For this review, use the dimensioned drawing (mm, ordinates from the lowest corner) and the shaded views. A direction names the side the tool comes from. Coordinates: 2 decimals unless noted, no trailing zeros. Loops run counter-clockwise (first coordinate to the right, second up) from the corner with the lowest first, then second, coordinate; pieces in that order, holes last. Notation, with made-up numbers: M 84.25,10.5 L 120.25,10.5 A18 cw 120.25,35.5 Z; hole C -2,17.5 d2. An arc over 180 degrees is marked long. Write item = value, one per line.
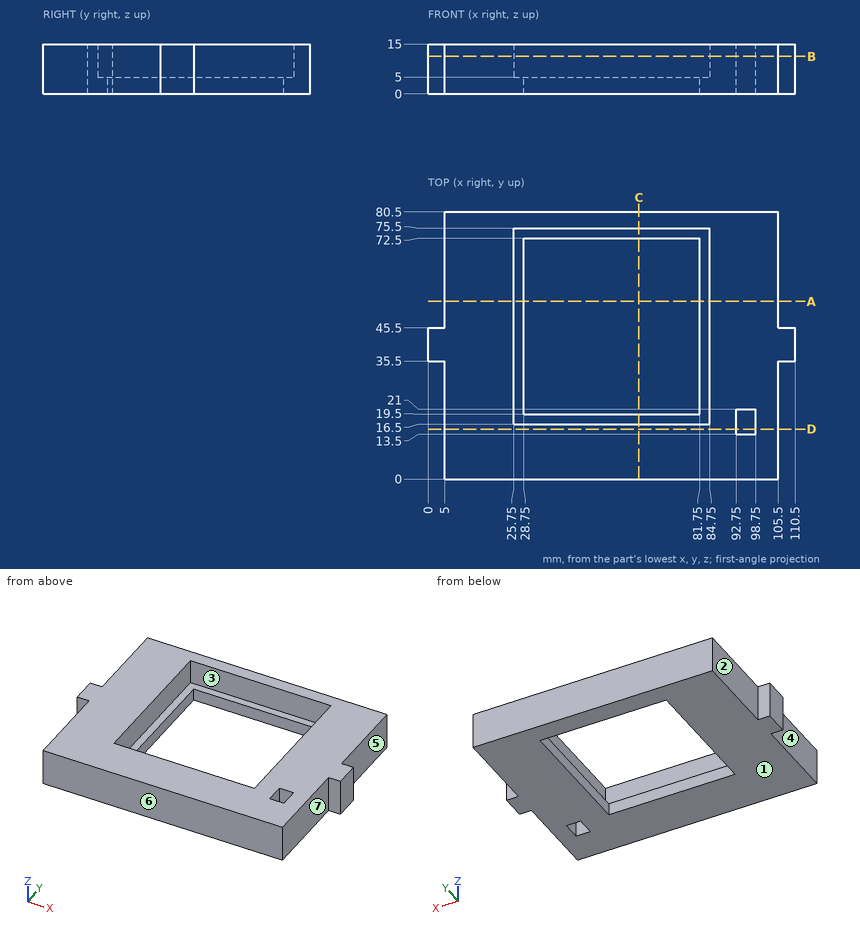
Q1. For pin 1 Ø4 at (x, z) = (1.5, 10.5) entering from -Y; pin 2 Ø5 at (y, z) = (53.5, 8) entering from +X; pin 3 Ø4 at (x, z) = (108.5, 8.5) entering from +Y, all flat-tipped, find the tip position at first contact; note any pin that passes through.
Solved:
pin_1 = 35.5
pin_2 = 105.5
pin_3 = 45.5
Q2. Machinability: for the marked faces 4, 5, 6 and 7, which of the approach directions +Z, -Z, +X, -X, +Y, -Y give a long, thin tool a straight path to every point of the face, cutting with its end or side? Answer none if there is none.
Solved:
face_4 = +Z, -Z, -X, -Y
face_5 = +Z, -Z, +X, +Y
face_6 = +Z, -Z, +X, -X, -Y
face_7 = +Z, -Z, +X, -Y
Q3. Add section B-B (z = 11.25). Write out the cut boundary in (x, y), and give its area (3 significant figures).
Solved:
outline = M 0,35.5 L 5,35.5 L 5,0 L 105.5,0 L 105.5,35.5 L 110.5,35.5 L 110.5,45.5 L 105.5,45.5 L 105.5,80.5 L 5,80.5 L 5,45.5 L 0,45.5 Z; hole M 25.75,16.5 L 84.75,16.5 L 84.75,75.5 L 25.75,75.5 Z; hole M 92.75,13.5 L 98.75,13.5 L 98.75,21 L 92.75,21 Z
area = 4,660 mm²
Q4. Add section C-C (x = 63.5). Write out the cut boundary in (y, z), and give its area (4 significant figures).
Solved:
outline = M 0,0 L 19.5,0 L 19.5,5 L 16.5,5 L 16.5,15 L 0,15 Z; M 72.5,0 L 80.5,0 L 80.5,15 L 75.5,15 L 75.5,5 L 72.5,5 Z
area = 352.5 mm²
Q5. For line 1 along Y through (x, z) = (37.5, 2.75); line 2 along Y through (x, z) = (41, 11); line 3 along X through (y, z) = (38, 12), list the stretches that pass through material, from the lowest coordinate up.
Solved:
line_1 = 0 to 19.5, 72.5 to 80.5
line_2 = 0 to 16.5, 75.5 to 80.5
line_3 = 0 to 25.75, 84.75 to 110.5
Q6. Add section A-A (y = 53.5). Write out the cut boundary in (x, z), and give its area (4 significant figures).
Solved:
outline = M 5,0 L 28.75,0 L 28.75,5 L 25.75,5 L 25.75,15 L 5,15 Z; M 81.75,0 L 105.5,0 L 105.5,15 L 84.75,15 L 84.75,5 L 81.75,5 Z
area = 652.5 mm²
Q7. Draft analysis for pull direction X (two halves, no side actions). For the marked faces 1, 2 and 3, state which applies: +X half, -X half, draft (parallel to the pull), parting line (faces both ways), or undercut.
Solved:
face_1 = draft
face_2 = -X half
face_3 = undercut
Q8. Add section D-D (y = 15). Write out the cut boundary in (x, z), and give its area (3 significant figures).
Solved:
outline = M 5,0 L 92.75,0 L 92.75,15 L 5,15 Z; M 98.75,0 L 105.5,0 L 105.5,15 L 98.75,15 Z
area = 1,420 mm²
